Geometry: see drawing. Coordinates: mm, zero at the bounding-box minimum. A direction names the side the tool comes from. Give positions to 0.01 mm unless a question says otherwise; leave off trailing zeros. Write each loop counter-clockwise with the first axis right and the second up, starting at its lowest first coordinate (ties: lowest second). Pieces come first, ordered by that corner, then holes. Notation, with made-up numbers: M -14,-23.75 L -4,-23.75 A15 cw -4,-1.75 Z; hole C 69.25,17 d1. An arc over 180 degrees is marked long. Use one line per item in the form item = value. Start each with the question number.
Item 1: Section query B-B on y = 13.5. Return loops of the section in (x, z) (1 decimal).
Item 2: Material intervals for line 1 along Y through (x, z) = (7, 0.55) (1 decimal); line 2 along Y through (x, z) = (5, 1.65) (1 decimal); line 3 along X through (y, z) = (11.25, 2.3) (1 decimal), sorted ascending. Write a range as from..to.
Item 3: Pull-direction query (Y, two-part tool) for the marked faces 3, 4 and 5; classes: released by +Y, released by -Y, zero draft, split by the parting line, or undercut.
Item 4: Access query for the marked faces 1 and 2. Directions: +Z, -Z, +X, -X, +Y, -Y. A direction counts if a zero-diameter tool reaches every point of the face in a straight line with its end or side. Return the directions, or none.
Item 5: Section query D-D on y = 3. Return loops of the section in (x, z).
Item 6: Section query C-C on x = 5. Return loops of the section in (y, z).
Item 7: Section query A-A on z = 1.9. Return loops of the section in (x, y) (1 decimal).
Item 8: Contact query for flat-ended pins moving along their axis: P1, Ø3, axis at x = 5, y = 11.82, coming from the -Z side; P2, Ø1.5, axis at x = 9.5, z = 0.5, coming from the -Y side (1 decimal); P3, Ø0.7, axis at y = 6, z = 2, coming from the +X side. Output: stop coordinate, or through.
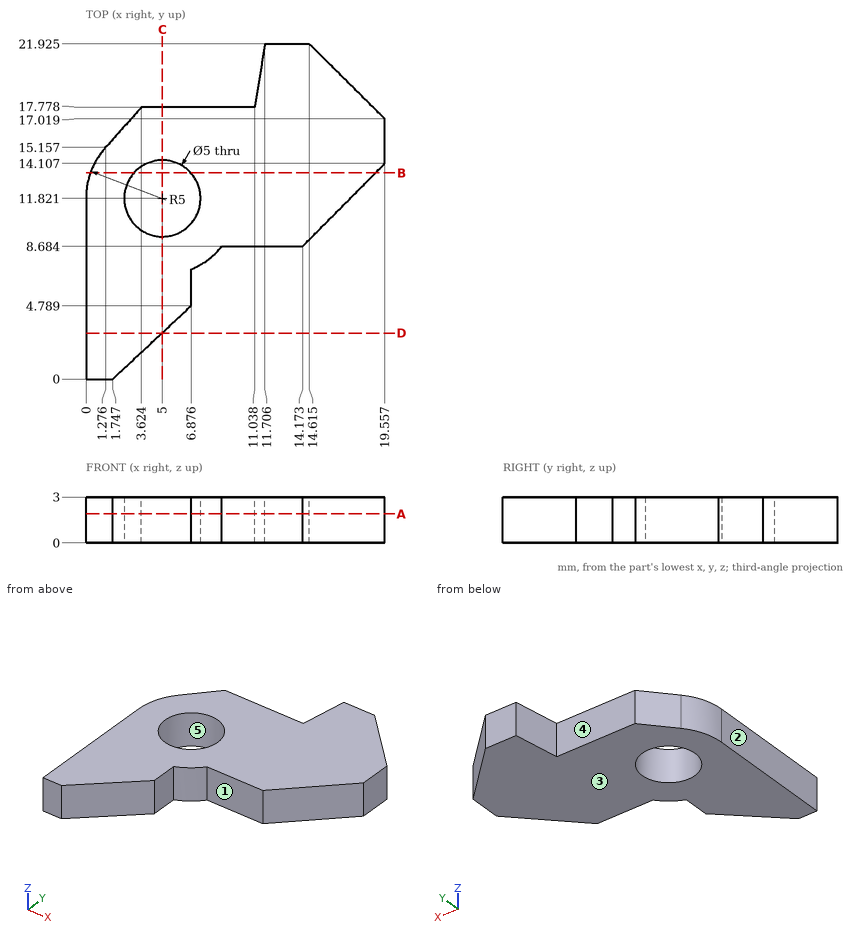
Answer sheet:
q1.outline = M 0.3,0 L 3.1,0 L 3.1,3 L 0.3,3 Z; M 6.9,0 L 19,0 L 19,3 L 6.9,3 Z
q2.line_1 = 7.2..10.3, 13.3..17.8
q2.line_2 = 3..9.3, 14.3..17.8
q2.line_3 = 0..2.6, 7.4..16.7
q3.face_3 = zero draft
q3.face_4 = released by +Y
q3.face_5 = undercut
q4.face_1 = +Z, -Z, +X, -Y
q4.face_2 = +Z, -Z, -X, +Y, -Y
q5.outline = M 0,0 L 4.96,0 L 4.96,3 L 0,3 Z
q6.outline = M 3.04,0 L 9.32,0 L 9.32,3 L 3.04,3 Z; M 14.32,0 L 17.78,0 L 17.78,3 L 14.32,3 Z
q7.outline = M 0,0 L 1.7,0 L 6.9,4.8 L 6.9,7.2 A5 ccw 8.9,8.7 L 14.2,8.7 L 19.6,14.1 L 19.6,17 L 14.6,21.9 L 11.7,21.9 L 11,17.8 L 3.6,17.8 L 1.3,15.2 A5 ccw 0,11.8 Z; hole C 5,11.8 d5
q8.P1 = through
q8.P2 = 8.5
q8.P3 = 6.88
